```python
from build123d import *

# Parameters (mm, degrees)
F0_W     = 80
F0_H     = 8
F0_R     = 1.75
F1_DEPTH = 3
F2_R     = 2


with BuildPart() as f1:
    # F0 (on Top) → F1 (new body)
    with BuildSketch(Plane.XY):
        Rectangle(F0_W, F0_H)
        with Locations((-35, 0)):
            Circle(F0_R, mode=Mode.SUBTRACT)
        Circle(F0_R, mode=Mode.SUBTRACT)
        with Locations((35, 0)):
            Circle(F0_R, mode=Mode.SUBTRACT)
    extrude(amount=F1_DEPTH)

    # F2
    f2_edges = [f1.edges().sort_by_distance(p)[0] for p in [
        (-40, -4, 1.5),
        (40, -4, 1.5),
        (40, 4, 1.5),
        (-40, 4, 1.5),
    ]]
    fillet(f2_edges, radius=F2_R)


solid = f1.part
```
Input: part model. Units: mm. Frame: model coordinates. Give positions to 0.01 mm unless a question says otherwise; leave off trailing zeros. Order: outer loops, then holes, each group sorted by start corner. A loop starts at its lowest first (then second) coordinate and runs counter-clockwise, first axis right, second up.
1. Pin query (flat end, axial travel): pin 1 Ø3 at (x, y) = (-35, 0) entering from +Z. Return the tip coordinate at first contact, or that it passes through.
Computed:
pin 1: passes through
2. Line query: probe 1 along Y at (x, z) = (0, 0.85); probe 2 along X at (y, z) = (1, 2.6); probe 3 along X at (y, z) = (1.5, 2.05). Output: solid intervals per line, ascending.
Computed:
probe 1: y = -4 to -1.75, 1.75 to 4
probe 2: x = -40 to -36.44, -33.56 to -1.44, 1.44 to 33.56, 36.44 to 40
probe 3: x = -40 to -35.9, -34.1 to -0.9, 0.9 to 34.1, 35.9 to 40
3. Cut plane C-C (x = 0). Return loops of the section in (y, z).
Computed:
outline: (-4, 0) - (-1.75, 0) - (-1.75, 3) - (-4, 3) - close; (1.75, 0) - (4, 0) - (4, 3) - (1.75, 3) - close
4. Draft query along Y for faces 1 (the face through (-39.43, -3.4, 1.52)), 2 (the face through (1.617, -0.67, 1.479)), 3 (the face through (-1, 2, 0)). Return one class per face: released by +Y, released by -Y, zero draft, split by the parting line, or undercut.
Computed:
face 1: released by -Y
face 2: undercut
face 3: zero draft
5. Cut plane A-A (y = 0). Return loops of the section in (x, z).
Computed:
outline: (-40, 0) - (-36.75, 0) - (-36.75, 3) - (-40, 3) - close; (-33.25, 0) - (-1.75, 0) - (-1.75, 3) - (-33.25, 3) - close; (1.75, 0) - (33.25, 0) - (33.25, 3) - (1.75, 3) - close; (36.75, 0) - (40, 0) - (40, 3) - (36.75, 3) - close
6. Cut plane B-B (z = 0.45). Return loops of the section in (x, y), and give its area (3 significant figures).
Computed:
outline: (-40, -2) arc R2 ccw to (-38, -4) - (38, -4) arc R2 ccw to (40, -2) - (40, 2) arc R2 ccw to (38, 4) - (-38, 4) arc R2 ccw to (-40, 2) - close; hole circle Ø3.5 at (-35, 0); hole circle Ø3.5 at (0, 0); hole circle Ø3.5 at (35, 0)
area: 608 mm2
